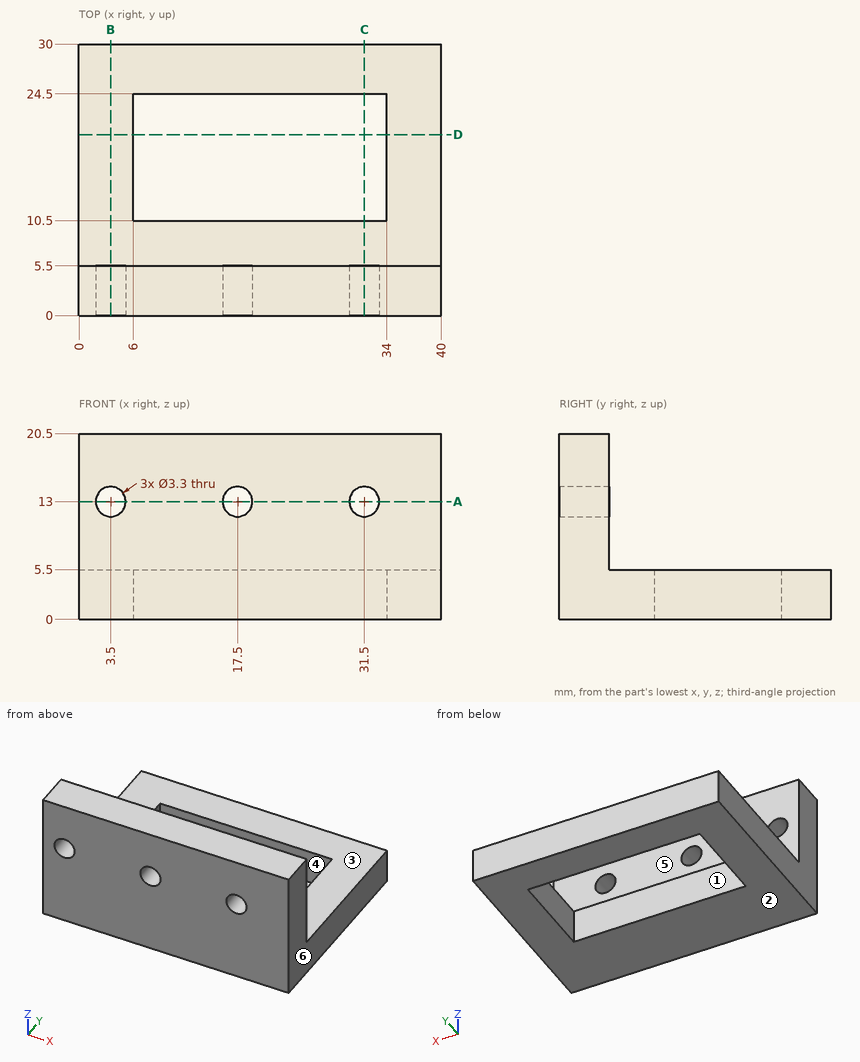
Verification items for this drawing (mm, ordinates from the low corner). A direction names the side the tool comes from. Round coordinates to 2 decimals unless told otherwise and drop trailing zeros. Order: outer loops, then holes, each group sorted by start corner. A loop starts at its lowest first (then second) coordinate and runs counter-clockwise, first axis right, second up. Notation, with made-up numbers: M 15.5,-29.5 L 61.5,-29.5 A25 ccw 61.5,-15.5 Z; hole C -15,-30.75 d1. An arc over 180 degrees is marked long. Answer in a Markdown table with one row per item. Add a question column.
Item 1: Sectioned sample at A-A, the plane z = 13. Enter the section's corners in (x, y), plus the area to 3 significant figures.
Item 2: Depth check by flat-ended pin: pin 1 Ø12 at (x, z) = (7, 15) entering from +Y; pin 2 Ø8 at (x, y) = (32.5, 22.5) entering from +Z. Enter the tip coordinate at first touch or a pass-through.
Item 3: Draft check along X on the marked faces 4, 5 and 6. Enter one of: released by +X, released by -X, zero draft, split by the parting line, or undercut.
Item 4: Material ranges on L1, parallel to X at y = 2.05, z = 13; L2, parallel to X at y = 13.75, z = 2; L3, parallel to Y at x = 13.5, z = 1.25, recorded low to high. Write a range as [from, to].
Item 5: Sectioned sample at B-B, the plane x = 3.5. Enter the section's corners in (y, z).
Item 6: Set-up check for the marked faces 1, 2 and 3: record each of +Z, -Z, +X, -X, +Y, -Y from which the full face is reachable in a straight line by a thin tool's end or side.
Item 7: Sectioned sample at C-C, the plane x = 31.5. Enter the section's corners in (y, z).
Item 8: Sectioned sample at D-D, the plane y = 20. Enter the section's corners in (x, z), plus the area to 3 significant figures.
Filled in:
| question | item | result |
|---|---|---|
| 1 | outline | M 0,0 L 1.85,0 L 1.85,5.5 L 0,5.5 Z; M 5.15,0 L 15.85,0 L 15.85,5.5 L 5.15,5.5 Z; M 19.15,0 L 29.85,0 L 29.85,5.5 L 19.15,5.5 Z; M 33.15,0 L 40,0 L 40,5.5 L 33.15,5.5 Z |
| 1 | area | 166 mm² |
| 2 | pin 1 | stops at y = 5.5 |
| 2 | pin 2 | stops at z = 5.5 |
| 3 | face 4 | undercut |
| 3 | face 5 | zero draft |
| 3 | face 6 | released by +X |
| 4 | L1 | x = [0, 1.85], [5.15, 15.85], [19.15, 29.85], [33.15, 40] |
| 4 | L2 | x = [0, 6], [34, 40] |
| 4 | L3 | y = [0, 10.5], [24.5, 30] |
| 5 | outline | M 0,0 L 30,0 L 30,5.5 L 5.5,5.5 L 5.5,11.35 L 0,11.35 Z; M 0,14.65 L 5.5,14.65 L 5.5,20.5 L 0,20.5 Z |
| 6 | face 1 | +Z, -Z |
| 6 | face 2 | -Z, +X, -X, +Y, -Y |
| 6 | face 3 | +Z, +X, -X, +Y |
| 7 | outline | M 0,0 L 10.5,0 L 10.5,5.5 L 5.5,5.5 L 5.5,11.35 L 0,11.35 Z; M 0,14.65 L 5.5,14.65 L 5.5,20.5 L 0,20.5 Z; M 24.5,0 L 30,0 L 30,5.5 L 24.5,5.5 Z |
| 8 | outline | M 0,0 L 6,0 L 6,5.5 L 0,5.5 Z; M 34,0 L 40,0 L 40,5.5 L 34,5.5 Z |
| 8 | area | 66.0 mm² |
